Autodesk Inventor part; units mm, degrees
ref_plane "Start Plane" through (0, 0, 0) normal (1, 0, 0) x (0, 1, 0)
ref_plane "XZ Plane" through (0, 0, 0) normal (0, 1, 0) x (-1, 0, 0)
ref_plane "XY Plane" through (0, 0, 0) normal (0, 0, 1) x (1, 0, 0)
sketch "Main Sketch" plane through (0, 0, 0) normal (0, 0, 1) x (1, 0, 0)
  line L0 (0, 0) -> (65, 0)
  line L1 (0, 0) -> (0, 3)
  line L2 (0, 3) -> (60, 3)
  line L3 (60, 3) -> (60, 4)
  line L4 (65, 4) -> (65, 0)
  line L5 (60, 4) -> (65, 4)
  dimension "d3" = 6
  dimension "d4" = 8
revolve "Revolution1" add sketch "Main Sketch" angle 360 about axis through (0, 0, 0) along (1, 0, 0)
chamfer "Chamfer1" distance 0.5 angle 45 1 edges at (0, -3, 0) measured on face at (40, 2.9903, -0.2414)
chamfer "Chamfer2" distance 0.5 angle 45 1 edges at (60, -4, 0) measured on face at (63.3333, 3.9482, -0.6416)
equation "\"Length\" = 65"
properties part number "Shaft" material "Steel"
Geometry: final body of the model. Coordinates: model frame, mm. A direction names the side the tool comes from. Give positions to 0.01 mm unless a question says otherwise; leave off trailing zeros. Write each loop counter-clockwise with the first axis right and the second up, starting at its lowest first coordinate (ties: lowest second). Pieces come first, ordered by that corner, then holes. Notation, with made-up numbers: (-38, -4) -> (-14, -4) arc R9 cw to (-14, 12) -> close; hole circle Ø1 at (31.25, 69.25). An arc over 180 degrees is marked (long way). Answer in a Markdown table with one row per item.
(1) Pin query (flat end, axial travel): pin 1 (4 mm diameter, centred on x = 10, z = 1.5, fed in from -Y); pin 2 (4 mm diameter, centred on x = 55.5, y = 2, fed in from +Z); pin 3 (1 mm diameter, centred on x = 50.5, z = 0.5, fed in from +Y). Return the tip coordinate at first contact, or that it passes through.
Answers below:
| item | result |
|---|---|
| pin 1 | y = -3 |
| pin 2 | z = 3 |
| pin 3 | y = 3 |
(2) Ray query, line 1 along X through (y, z) = (-1.75, 2.75); line 2 along Y through (x, z) = (62.5, -0.25); line 3 along Z through (x, y) = (49.5, 0). Return the intervals inside material, ascending. Write a range as [from, to].
Answers below:
| item | result |
|---|---|
| line 1 | [60, 65] |
| line 2 | [-3.99, 3.99] |
| line 3 | [-3, 3] |
(3) Section query C-C on x = 7. Return loops of the section in (y, z), then the cut area to 3 significant figures.
Answers below:
| item | result |
|---|---|
| outline | circle Ø6 at (0, 0) |
| area | 28.3 mm^2 |
(4) Set-up query: faces 1 (the flat face through (0, 0, 0)), 2 (the flat face through (60, 3, 1)). Return all of +Z, -Z, +X, -X, +Y, -Y with unobstructed straight access to the full face (end or side cutting, diameter ignored); none if empty.
Answers below:
| item | result |
|---|---|
| face 1 | +Z, -Z, -X, +Y, -Y |
| face 2 | -X |
(5) Section query A-A on y = 0. Return loops of the section in (x, z), then the cut area to 4 significant figures.
Answers below:
| item | result |
|---|---|
| outline | (0, -2.5) -> (0.5, -3) -> (60, -3) -> (60, -3.5) -> (60.5, -4) -> (65, -4) -> (65, 4) -> (60.5, 4) -> (60, 3.5) -> (60, 3) -> (0.5, 3) -> (0, 2.5) -> close |
| area | 399.5 mm^2 |
